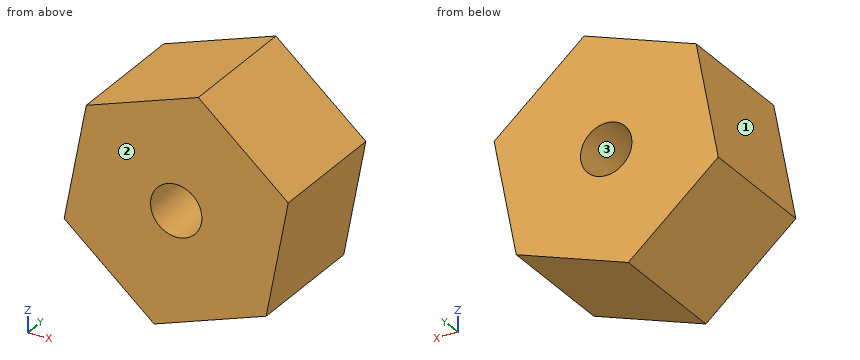
Autodesk Inventor part; units mm, degrees
ref_plane "YZ Plane" through (0, 0, 0) normal (1, 0, 0) x (0, 1, 0)
ref_plane "XZ Plane" through (0, 0, 0) normal (0, 1, 0) x (-1, 0, 0)
ref_plane "XY Plane" through (0, 0, 0) normal (0, 0, 1) x (1, 0, 0)
sketch "Szkic1" plane through (0, 0, 0) normal (0, 1, 0) x (-1, 0, 0)
  line L0 (0.8601, -4.538) -> (-3.5, -3.0139)
  line L1 (-3.5, -3.0139) -> (-4.3601, 1.5242)
  line L2 (-4.3601, 1.5242) -> (-0.8601, 4.538)
  line L3 (-0.8601, 4.538) -> (3.5, 3.0139)
  line L4 (3.5, 3.0139) -> (4.3601, -1.5242)
  line L5 (4.3601, -1.5242) -> (0.8601, -4.538)
  point P0 (0, 0)
  point P1 (0, 0)
  dimension "d0" = 4
  dimension "d1" = 3.5
extrude "Wyciągnięcie proste1" add sketch "Szkic1" along normal blind 5
sketch "Szkic2" plane through (0, 5, 0) normal (0, 1, 0) x (1, 0, 0)
  circle A0 centre (0, 0) radius 1
  dimension "d4" = 2
extrude "Wyciągnięcie proste2" cut sketch "Szkic2" against normal blind 5
thread "Gwint1"
properties part number "nakretka_m2"
The model under review builds one solid part; all positions refer to its coordinate system, in mm. Face numbers are marked on the shaded views. Round coordinates to 2 decimals unless told otherwise and drop trailing zeros. Loops run counter-clockwise (first coordinate to the right, second up) from the corner with the lowest first, then second, coordinate; pieces in that order, holes last. Notation, with made-up numbers: (-1, 46.5) -> (39, 46.5) arc R17 ccw to (39, 79.5) -> close; hole circle Ø1 at (31.25, 89). An arc over 180 degrees is marked (long way). Answer as a JSON object with one key per item and string values. Group by question number.
1) We need section C-C on x = 0. Write out the cut boundary in (y, z), then the cut area to 3 significant figures.
2) We need section A-A on y = 4.4. Write out the cut boundary in (x, z), then the cut area to 3 significant figures.
3) We need section D-D on x = 1.25. Write out the cut boundary in (y, z).
4) Mouldability with a two-part tool opening along X and no side actions: class the marked faces 1, 2 and 3 as released by +X, released by -X, zero draft, split by the parting line, or undercut.
5) For pin 1 Ø2 at (x, y) = (-0.5, 3.5) entering from +Z; pin 2 Ø1.5 at (y, z) = (2, -1) entering from +X, all flat-tipped, find the tip position at first contact; note any pin that passes through.
6) We need section B-B on z = 0. Write out the cut boundary in (x, y).
7) For line 1 (X direction, y = 3.95, z = 0); line 2 (Z direction, x = 0, y = 3.6); line 3 (X direction, y = 1.4, z = 0.25), list the stretches that pass through material, from the lowest coordinate up. Write a range as [from, to].
Result set:
{
 "1": {"outline": "(0, -4.24) -> (5, -4.24) -> (5, -1) -> (0, -1) -> close; (0, 1) -> (5, 1) -> (5, 4.24) -> (0, 4.24) -> close", "area": "32.4 mm²"},
 "2": {"outline": "(-4.36, -1.52) -> (-0.86, -4.54) -> (3.5, -3.01) -> (4.36, 1.52) -> (0.86, 4.54) -> (-3.5, 3.01) -> close; hole circle Ø2 at (0, 0)", "area": "52.3 mm²"},
 "3": {"outline": "(0, -3.8) -> (5, -3.8) -> (5, 4.2) -> (0, 4.2) -> close"},
 "4": {"face 1": "released by -X", "face 2": "zero draft", "face 3": "undercut"},
 "5": {"pin 1": "z = 4.41", "pin 2": "x = 4.02"},
 "6": {"outline": "(-4.07, 0) -> (-1, 0) -> (-1, 5) -> (-4.07, 5) -> close; (1, 0) -> (4.07, 0) -> (4.07, 5) -> (1, 5) -> close"},
 "7": {"line 1": "[-4.07, -1], [1, 4.07]", "line 2": "[-4.24, -1], [1, 4.24]", "line 3": "[-4.02, -0.97], [0.97, 4.12]"}
}
